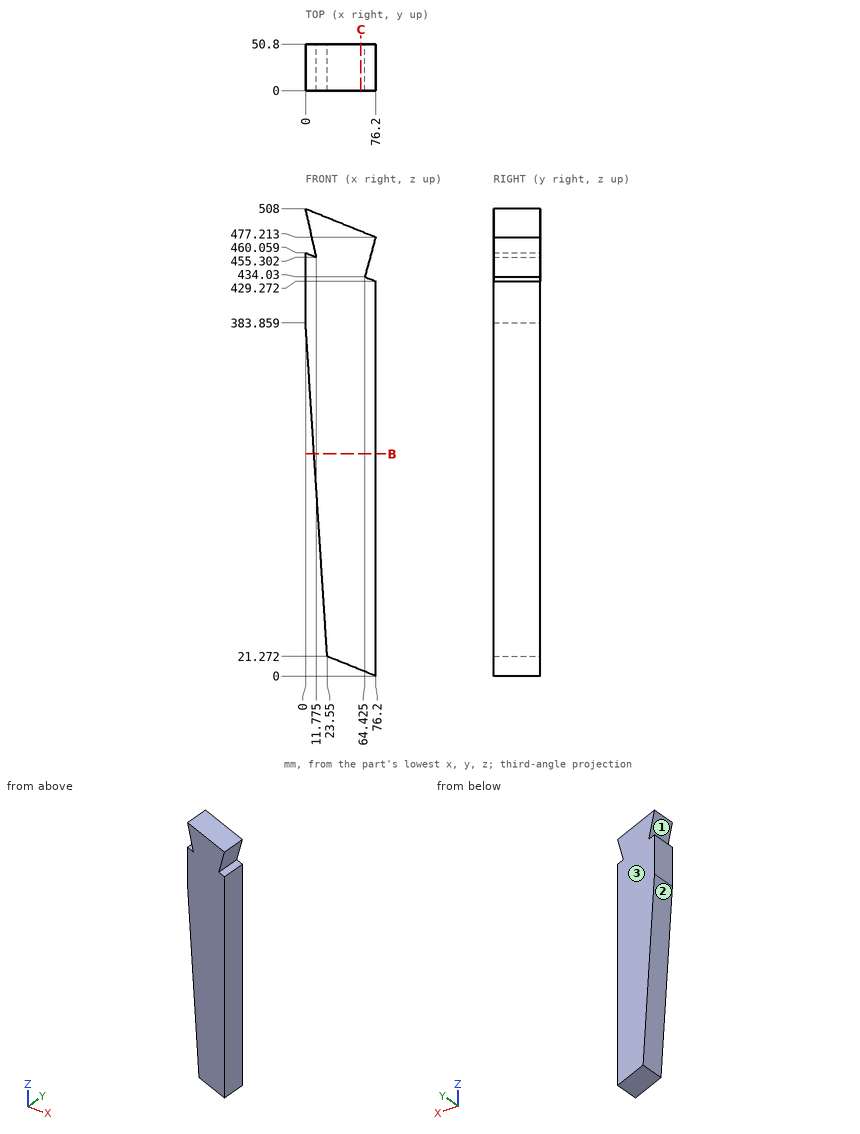
The figure shows three views and two pictorial views of one solid part (mm, origin at its lowest corner). Answer the questions. Round coordinates to 2 decimals unless told otherwise and drop trailing zeros. Write each loop counter-clockwise with the first axis right and the second up, starting at its lowest first coordinate (ties: lowest second). Pieces come first, ordered by that corner, then holes. Notation, with made-up numbers: M 31,57 L 86,57 A22 cw 86,78 Z; hole C 12.5,53.5 d6. An arc over 180 degrees is marked long. Write each question's results on one line, items separated by ' | '. Start each with the question number.
(1) The part is cut by section C-C, the plane x = 60. Write down the section's boundary in (y, z) (1 decimal), and give its area (3 significant figures).
(2) Determine the mould class of the marked faces 1, 2 and 3 for opening direction Z: +Z half, -Z half, draft (parallel to the pull), parting line (faces both ways), or undercut.
(3) Find the intervals of material crossed by line 1 (X direction, y = 12, z = 83); line 2 (X direction, y = 9, z = 102); line 3 (Z direction, x = 44, y = 30), in increasing order.
(4) The part is cut by section B-B, the plane z = 241.5. Write down the section's boundary in (x, y), and give its area (3 significant figures).
(5) Each of these flat-tipped pins is pushed along its axis until it touches: P1, Ø12, axis at y = 6, z = 373, coming from the -X side; P2, Ø10, axis at y = 22, z = 94.5, coming from the -X side; P3, Ø5, axis at y = 13.5, z = 78.5, coming from the -X side. Where does it stop, or does it pass through?
Worked answers:
1) outline: M 0,6.5 L 50.8,6.5 L 50.8,483.8 L 0,483.8 Z | area: 24,200 mm²
2) face 1: undercut | face 2: -Z half | face 3: draft
3) line 1: x = 19.54 to 76.2 | line 2: x = 18.31 to 76.2 | line 3: z = 13.01 to 490.22
4) outline: M 9.25,0 L 76.2,0 L 76.2,50.8 L 9.25,50.8 Z | area: 3,400 mm²
5) P1: stops at x = 0.32 | P2: stops at x = 18.47 | P3: stops at x = 19.67
